Check sheet for the drawn part. Datum: minimum x, y, z corner. Units: mm. Give positions to 0.01 mm unless a question says otherwise; leave off trailing zeros. Loops run counter-clockwise (first coordinate to the right, second up) from the corner with the lowest first, then second, coordinate; pieces in that order, holes last. Notation, with made-up numbers: (45.25, 48.25) - (94.25, 48.25) arc R24 ccw to (94.25, 76.25) - close; hole circle Ø3 at (23.5, -25.5). An arc over 180 degrees is marked (long way). Use one line per item in the form item = value.
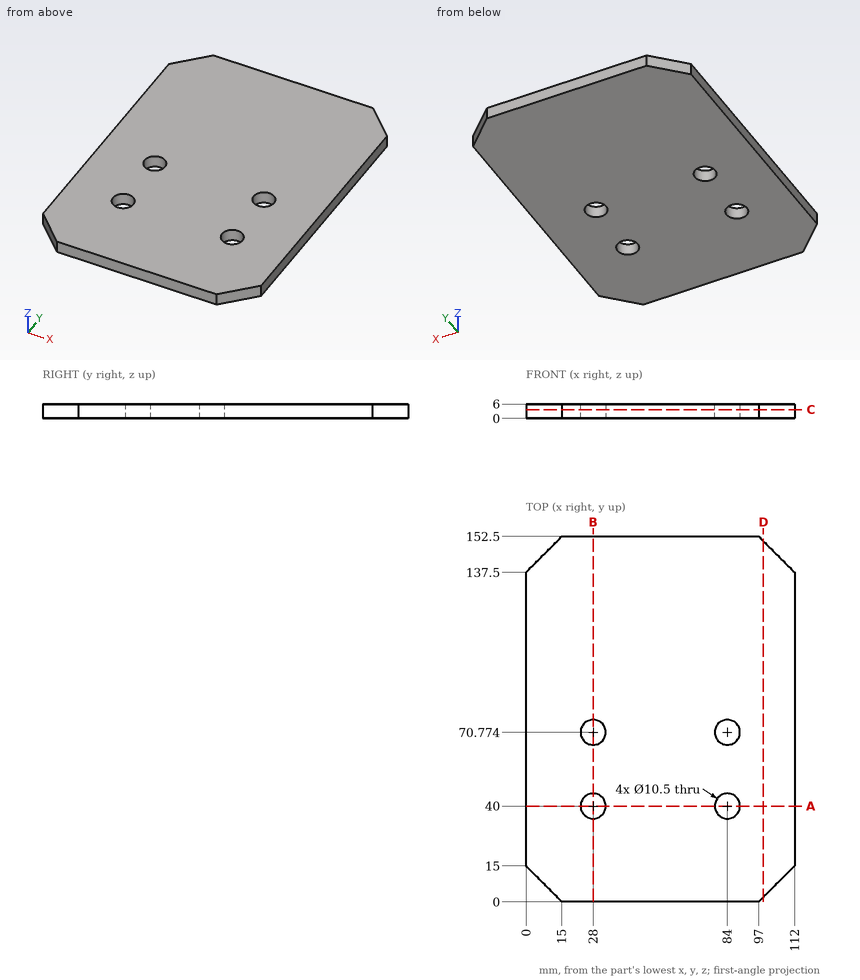
1. Section check C-C, the plane z = 3.7. Record the cut outline in (x, y), then the cut area to 3 significant figures.
Result set:
outline = (0, 15) - (15, 0) - (97, 0) - (112, 15) - (112, 137.5) - (97, 152.5) - (15, 152.5) - (0, 137.5) - close; hole circle Ø10.5 at (28, 40); hole circle Ø10.5 at (28, 70.77); hole circle Ø10.5 at (84, 40); hole circle Ø10.5 at (84, 70.77)
area = 16,300 mm²
2. Scan lines: probe 1 along Y at (x, z) = (84, 4.5); probe 2 along X at (y, z) = (68, 0.3); probe 3 along X at (y, z) = (72.5, 3.15). Record each from-to range of solid material in increasing order.
Result set:
probe_1 = 0 to 34.75, 45.25 to 65.52, 76.02 to 152.5
probe_2 = 0 to 23.54, 32.46 to 79.54, 88.46 to 112
probe_3 = 0 to 23.04, 32.96 to 79.04, 88.96 to 112
3. Section check A-A, the plane y = 40. Record the cut outline in (x, z), then the cut area to 3 significant figures.
Result set:
outline = (0, 0) - (22.75, 0) - (22.75, 6) - (0, 6) - close; (33.25, 0) - (78.75, 0) - (78.75, 6) - (33.25, 6) - close; (89.25, 0) - (112, 0) - (112, 6) - (89.25, 6) - close
area = 546 mm²
4. Section check D-D, the plane x = 99. Record the cut outline in (y, z), then the cut area to 3 significant figures.
Result set:
outline = (2, 0) - (150.5, 0) - (150.5, 6) - (2, 6) - close
area = 891 mm²
5. Depth check by flat-ended pin: pin 1 Ø1.5 at (x, z) = (99.5, 4.5) entering from +Y. Enter the tip coordinate at first touch or a pass-through.
Result set:
pin_1 = 150.75
6. Section check B-B, the plane x = 28. Record the cut outline in (y, z).
Result set:
outline = (0, 0) - (34.75, 0) - (34.75, 6) - (0, 6) - close; (45.25, 0) - (65.52, 0) - (65.52, 6) - (45.25, 6) - close; (76.02, 0) - (152.5, 0) - (152.5, 6) - (76.02, 6) - close
